Geometry: final body of the model. Coordinates: model frame, mm. Give positions to 0.01 mm unless a question says otherwise; leave off trailing zeros. Write each loop counter-clockwise with the first axis right and the second up, starting at its lowest first coordinate (ties: lowest second). Pieces come first, ordered by that corner, then holes. Notation, with made-up numbers: M 88,-36 L 112,-36 A28 ccw 112,-2 Z; hole C 22,-11.75 d4. An arc over 180 degrees is marked long. Use one line per item in the form item = value. Start each with the question number.
Item 1: Section query D-D on y = 93.5. Return loops of the section in (x, z), then the cut area to 3 significant figures.
Item 2: Section query A-A on x = -38.5. Return loops of the section in (y, z).
Item 3: Section query B-B on z = -1. Return loops of the section in (x, y).
Item 4: Pull-direction query (Y, two-part tool) for faces 1 (the cylindrical face through (-34.41, 71.2, -1.48)), 2 (the flat face through (40, 51, -1)), 3 (the cylindrical face through (-71.484, 69.929, -1.479)); classes: released by +Y, released by -Y, zero draft, split by the parting line, or undercut.
Item 5: Contact query for a flat-ended pin moving along its axis: P1, Ø9, axis at x = -37.1, y = 66.98, coming from the +Z side. Output: stop coordinate, or through.
Item 6: Material intervals for line 1 along X through (y, z) = (51.5, -1.8); line 2 along Y through (x, z) = (-41, -1); line 3 along Y through (x, z) = (-54.5, -1.85), sorted ascending. Write a range as from..to.
Item 7: Section query C-C on y = 20. Return loops of the section in (x, z), then the cut area to 3 significant figures.
from build123d import *

# Parameters (mm, degrees)
ESBO_O1_R          = 5
FLANGE_BASE1_DEPTH = 3


# Sheet-metal steps are written as plain solids
with BuildPart() as part:
    # Esboço1 → Flange-base1 (new body)
    with BuildSketch(Plane.XY):
        with BuildLine():
            Line((0, 0), (-100, 0))
            ThreePointArc((-100, 0), (-70.710678119, 70.710678119), (0, 100))
            Line((0, 100), (40, 100))
            Line((40, 100), (40, 0))
            Line((40, 0), (0, 0))
        make_face()
        with Locations((-20, 20)):
            Circle(ESBO_O1_R, mode=Mode.SUBTRACT)
        with Locations((-55.355339059, 55.355339059)):
            Circle(ESBO_O1_R, mode=Mode.SUBTRACT)
        with Locations((-37.101007166, 66.984631039)):
            Circle(ESBO_O1_R, mode=Mode.SUBTRACT)
        with Locations((-15.642212863, 69.809734905)):
            Circle(ESBO_O1_R, mode=Mode.SUBTRACT)
    extrude(amount=-FLANGE_BASE1_DEPTH)


solid = part.part
Answer sheet:
q1.outline = M -35.46,-3 L 40,-3 L 40,0 L -35.46,0 Z
q1.area = 226 mm2
q2.outline = M 0,-3 L 62.18,-3 L 62.18,0 L 0,0 Z; M 71.78,-3 L 92.29,-3 L 92.29,0 L 71.78,0 Z
q3.outline = M -100,0 L 40,0 L 40,100 L 0,100 A100 ccw Z; hole C -55.36,55.36 d10; hole C -37.1,66.98 d10; hole C -20,20 d10; hole C -15.64,69.81 d10
q4.face_1 = undercut
q4.face_2 = zero draft
q4.face_3 = released by +Y
q5.P1 = through
q6.line_1 = -85.72..-58.54, -52.17..40
q6.line_2 = 0..63.85, 70.11..91.21
q6.line_3 = 0..50.43, 60.28..83.84
q7.outline = M -97.98,-3 L -25,-3 L -25,0 L -97.98,0 Z; M -15,-3 L 40,-3 L 40,0 L -15,0 Z
q7.area = 384 mm2
